Source: CAD feature listing. Evaluate the final solid. Frame: model axes, mm. A direction names the side the tool comes from. Give positions to 0.01 mm unless a question says otherwise; leave off trailing zeros. Write each loop counter-clockwise with the first axis right and the second up, starting at its lowest first coordinate (ties: lowest second). Pieces come first, ordered by that corner, then holes. Notation, with made-up numbers: (85.25, 73.5) -> (98.25, 73.5) arc R13 cw to (98.25, 82.5) -> close; hole circle Ø4 at (-31.75, 48.5). An arc over 180 degrees is marked (long way). Write item = value, one per line.
from build123d import *

# Parameters (mm, degrees)
EXTRUDE_1_DEPTH = 2
EXTRUDE_2_DEPTH = 4
SHELL_START     = -4
SHELL_4_DEPTH   = 2


with BuildPart() as part:
    # 草图1 → 凸台-拉伸1 (new body)
    with BuildSketch(Plane(origin=(0, 0, 0), x_dir=(1, 0, 0), z_dir=(0, 1, 0))):
        Polygon((-100, -133.049582772), (-36, -170), (36, -170), (100, -133.049582772), (100, -72), (68, -72), (68, 0), (-68, 0), (-68, -72), (-100, -72), align=None)
    extrude(amount=EXTRUDE_1_DEPTH)

    # 草图2 → 凸台-拉伸2 (add)
    with BuildSketch(Plane(origin=(0, 0, 0), x_dir=(1, 0, 0), z_dir=(0, 1, 0))):
        Polygon((95.8, -76.2), (63.8, -76.2), (63.8, -4.2), (-63.8, -4.2), (-63.8, -76.2), (-95.8, -76.2), (-95.8, -130.624711641), (-34.874613392, -165.8), (34.874613392, -165.8), (95.8, -130.624711641), align=None)
    extrude(amount=-EXTRUDE_2_DEPTH)

    # 抽壳4: read off the stored shape, not the designer's step
    # 抽壳4 outline → 抽壳4 (cut)
    with BuildSketch(Plane(origin=(0, 0, 0), x_dir=(1, 0, 0), z_dir=(0, 1, 0)).offset(SHELL_START)):
        Polygon((33.802816622, -161.8), (91.8, -128.315310565), (91.8, -80.2), (59.8, -80.2), (59.8, -8.2), (-59.8, -8.2), (-59.8, -80.2), (-91.8, -80.2), (-91.8, -128.315310565), (-33.802816622, -161.8), align=None)
    extrude(amount=SHELL_4_DEPTH, mode=Mode.SUBTRACT)


solid = part.part
1) Contact query for flat-ended pins moving along their axis: pin 1 (3 mm diameter, centred on x = -4, y = -2.5, fed in from -Z); pin 2 (2 mm diameter, centred on x = 52, y = -2.5, fed in from +Z); pin 3 (1 mm diameter, centred on y = 1, z = 34.5, fed in from +X). Output: stop coordinate, or through.
Computed:
pin_1 = 4.2
pin_2 = 156.49
pin_3 = 68
2) Material intervals for L1, parallel to X at y = -2.65, z = 74; L2, parallel to X at y = -2.4, z = 116; L3, parallel to X at y = -0.6, z = 50, sorted ascending.
Computed:
L1 = -63.8 to -59.8, 59.8 to 63.8
L2 = -95.8 to -91.8, 91.8 to 95.8
L3 = -63.8 to 63.8
3) Cut plane A-A (y = -3.1). Return the cut outline in (x, z).
Computed:
outline = (-95.8, 76.2) -> (-63.8, 76.2) -> (-63.8, 4.2) -> (63.8, 4.2) -> (63.8, 76.2) -> (95.8, 76.2) -> (95.8, 130.62) -> (34.87, 165.8) -> (-34.87, 165.8) -> (-95.8, 130.62) -> close; hole (-91.8, 80.2) -> (-59.8, 80.2) -> (-59.8, 8.2) -> (59.8, 8.2) -> (59.8, 80.2) -> (91.8, 80.2) -> (91.8, 128.32) -> (33.8, 161.8) -> (-33.8, 161.8) -> (-91.8, 128.32) -> close
4) Cut plane C-C (x = -4). Return the cut outline in (y, z).
Computed:
outline = (-4, 4.2) -> (0, 4.2) -> (0, 0) -> (2, 0) -> (2, 170) -> (0, 170) -> (0, 165.8) -> (-4, 165.8) -> (-4, 161.8) -> (-2, 161.8) -> (-2, 8.2) -> (-4, 8.2) -> close
5) Cut plane B-B (z = 60). Return the cut outline in (x, y).
Computed:
outline = (-68, 0) -> (-63.8, 0) -> (-63.8, -4) -> (-59.8, -4) -> (-59.8, -2) -> (59.8, -2) -> (59.8, -4) -> (63.8, -4) -> (63.8, 0) -> (68, 0) -> (68, 2) -> (-68, 2) -> close
6) Draft query along Z for faces 1 (the flat face through (80, -2, 76.2)), 2 (the flat face through (-1, -2, 84)), 3 (the flat face through (62.4, -3.01, 145.29)), 4 (the flat face through (0, -2, 165.8)). Return one class per face: pulls with the +Z half, pulls with the -Z half, needs draft (parallel to the pull), parting line crosses it, or undercut.
Computed:
face_1 = pulls with the -Z half
face_2 = undercut
face_3 = undercut
face_4 = pulls with the +Z half
7) Access query for faces 5 (the flat face through (95.8, -2, 104)), 6 (the flat face through (1, -2, 4.2)), 7 (the flat face through (-95.8, -2, 103)), 8 (the flat face through (-63.21, -3.01, 144.82)). Directions: +Z, -Z, +X, -X, +Y, -Y. A direction counts if a zero-diameter tool reaches every point of the face in a straight line with its end or side. Return the directions, or none.
Computed:
face_5 = +Z, -Z, +X, -Y
face_6 = -Z, +X, -X, -Y
face_7 = +Z, -Z, -X, -Y
face_8 = -Y
